Could you check a few things on this model? Use its own coordinates, in mm. A direction names the side the tool comes from. Coordinates: 2 decimals unless noted, no trailing zeros. Order: outer loops, then holes, each group sorted by start corner. A loop starts at its lowest first (then second) coordinate and runs counter-clockwise, first axis right, second up. Notation, with made-up numbers: (-29, 28) - (-3, 28) arc R25 cw to (-3, 58) - close; hole circle Ø4 at (73, 4). An arc over 180 degrees is marked (long way). Answer as a JSON object with one key per item and string values. Group by question number.
(1) Please list where these lines run through material, in increasing order: probe 1 along Y at (x, z) = (0, 4.5); probe 2 along Y at (x, z) = (0, 6.85); probe 3 along Z at (x, y) = (6, 1).
(2) Will these pins go through, and if not, where does the flat tip stop? P1, Ø14.5, axis at x = 0, y = 0, coming from the +Z side; P2, Ø5, axis at x = -4.5, z = 8.5, coming from the +Y side; P3, Ø2, axis at y = -2, z = 6.5, coming from the -X side.
(3) Imagine slicing it at A-A, the plane x = 0. Write out the boundary of the cut face in (y, z), and give its area (3 significant figures).
(4) Which directions (+Z, -Z, +X, -X, +Y, -Y) give clear straight access to the entire face, cutting with the end or side of a thin tool? Please do faces 1 (the flat face through (0, 0, 0)), 2 (the flat face through (0, 0, 4)).
(5) We'd pull the mould along Y, two halves only. Please class faces 3 (the cylindrical face through (2.124, -9.567, 5.014)), 4 (the cylindrical face through (1.172, 8.923, 7.521)), 5 (the flat face through (-3, 10, 10)), 6 (the cylindrical face through (14.985, 0.66, 4.944)): pulls with the +Y half, pulls with the -Y half, needs draft (parallel to the pull), parting line crosses it, or undercut.
(6) Imagine slicing it at C-C, the plane z = 3. Write out the boundary of the cut face in (x, y).
from build123d import *

# Parameters (mm, degrees)
F2_R = 1
F3_R = 1
F4_R = 1


with BuildPart() as f1:
    # F0 (on Front) → F1 (revolve)
    with BuildSketch(Plane.XZ):
        Polygon((-15, 0), (0, 0), (0, 4), (-9.8, 4), (-9.8, 6), (-9, 6), (-9, 10), (-15, 10), align=None)
    revolve(axis=Axis((0, 0, 2), (0, 0, -1)))

    # F2
    f2_edges = [f1.edges().sort_by_distance(p)[0] for p in [
        (15, 0, 10),
    ]]
    fillet(f2_edges, radius=F2_R)

    # F3
    f3_edges = [f1.edges().sort_by_distance(p)[0] for p in [
        (9, 0, 10),
    ]]
    fillet(f3_edges, radius=F3_R)

    # F4
    f4_edges = [f1.edges().sort_by_distance(p)[0] for p in [
        (15, 0, 0),
    ]]
    fillet(f4_edges, radius=F4_R)


solid = f1.part
Result set:
{
 "1": {"probe 1": "y = -15 to -9.8, 9.8 to 15", "probe 2": "y = -15 to -9, 9 to 15", "probe 3": "z = 0 to 4"},
 "2": {"P1": "stops at z = 4", "P2": "stops at y = 14.87", "P3": "stops at x = -14.97"},
 "3": {"outline": "(-15, 1) arc R1 ccw to (-14, 0) - (14, 0) arc R1 ccw to (15, 1) - (15, 9) arc R1 ccw to (14, 10) - (10, 10) arc R1 ccw to (9, 9) - (9, 6) - (9.8, 6) - (9.8, 4) - (-9.8, 4) - (-9.8, 6) - (-9, 6) - (-9, 9) arc R1 ccw to (-10, 10) - (-14, 10) arc R1 ccw to (-15, 9) - close", "area": "188 mm^2"},
 "4": {"face 1": "-Z, +X, -X, +Y, -Y", "face 2": "none"},
 "5": {"face 3": "undercut", "face 4": "undercut", "face 5": "needs draft", "face 6": "parting line crosses it"},
 "6": {"outline": "circle Ø30 at (0, 0)"}
}
